Verification items for the finished model (mm, model axes). A direction names the side the tool comes from. Coordinates: 2 decimals unless noted, no trailing zeros. Order: outer loops, then holes, each group sorted by start corner. A loop starts at its lowest first (then second) coordinate and runs counter-clockwise, first axis right, second up. Notation, with made-up numbers: (-10.75, -9.5) -> (39.25, -9.5) arc R24 ccw to (39.25, 15.5) -> close; hole circle Ø3 at (-30, 2). An arc over 180 degrees is marked (long way). Write item = value, one per line. Start each with the question number.
1. Cross-section at C-C on z = 40.5. Record the cut outline in (x, y) (3 decimals).
2. Cross-section at B-B on z = 15.5. Record the cut outline in (x, y), plus the area to 3 significant figures.
3. Cross-section at A-A on y = -50.8. Record the cut outline in (x, z) (3 decimals).
4. Set-up check for faces 4 (the cylindrical face through (30.904, -11.269, 7.96)), 5 (the cylindrical face through (92.25, -88.18, 3.13)), 6 (the flat face through (61.925, -50, 32)): record each of +Z, -Z, +X, -X, +Y, -Y from which the full face is reachable in a straight line by a thin tool's end or side.
5. Go/stop test with flat-tipped pins: P1, Ø3, axis at x = 95.5, y = -91, coming from the +Z side; P2, Ø5, axis at y = -46.5, z = 41.5, coming from the +X side; P3, Ø10, axis at y = -50.8, z = 46.355, coming from the -X side; P4, Ø4, axis at y = -50.8, z = 46.355, coming from the -X side. Record where each tip stops, or that it passes through.
6. Thickness scan on line 1 along X through (y, z) = (-76.5, 32); line 2 along X through (y, z) = (-12, 4). Record the ranges inside material, lowest first. Write a range as from..to.
7. Release check for a two-part mould opening along Y. For faces 1 (the flat face through (54.019, -22.536, 44.761)), 2 (the flat face through (26, -50, 9.525)), 3 (the flat face through (92, -90, 6.35)) record: +Y half, -Y half, draft (parallel to the pull), parting line (faces both ways), or undercut.
8. Cross-section at D-D on x = 103. Record the cut outline in (y, z) (3 decimals).
from build123d import *

# Parameters (mm, degrees)
F1_DEPTH       = 101.6
F3_D           = 4.7752
F3_CBORE_D     = 9.525
F3_CBORE_DEPTH = 3.175
F5_D           = 4.7752
F5_CBORE_D     = 9.525
F5_CBORE_DEPTH = 3.175
F7_D           = 6.35
F8_SIZE        = 44.45
F9_R           = 12.7


with BuildPart() as f1:
    # F0 (on Front) → F1 (new body)
    with BuildSketch(Plane.XZ):
        Polygon((0, 9.525), (0, 0), (119.0752, 0), (119.0752, 9.525), (68.2752, 9.525), (68.2752, 66.675), (61.9252, 66.675), (61.9252, 9.525), (57.15, 9.525), (57.15, 66.675), (50.8, 66.675), (50.8, 9.525), align=None)
    extrude(amount=F1_DEPTH)

    # F3 (through all)
    with Locations(Plane.XY.offset(9.525)):
        with Locations((26.361667, -12.7), (26.361667, -88.9)):
            CounterBoreHole(F3_D / 2, F3_CBORE_D / 2, F3_CBORE_DEPTH)

    # F5 (through all)
    with Locations(Plane.XY.offset(9.525)):
        with Locations((94.527818, -12.7), (94.527818, -88.9)):
            CounterBoreHole(F5_D / 2, F5_CBORE_D / 2, F5_CBORE_DEPTH)

    # F7 (through all)
    with Locations(Plane(origin=(50.8, 0, 0), x_dir=(0, -1, 0), z_dir=(-1, 0, 0))):
        with Locations((50.8, 46.355)):
            Hole(F7_D / 2)

    # F8
    f8_edges = [f1.edges().sort_by_distance(p)[0] for p in [
        (53.975, 0, 66.675),
        (53.975, -101.6, 66.675),
        (65.1002, 0, 66.675),
        (65.1002, -101.6, 66.675),
    ]]
    chamfer(f8_edges, length=F8_SIZE)

    # F9
    f9_edges = [f1.edges().sort_by_distance(p)[0] for p in [
        (0, 0, 4.7625),
        (0, -101.6, 4.7625),
        (119.0752, -101.6, 4.7625),
        (119.0752, 0, 4.7625),
    ]]
    fillet(f9_edges, radius=F9_R)


solid = f1.part
Worked out:
q1.outline = (50.8, -83.325) -> (57.15, -83.325) -> (57.15, -18.275) -> (50.8, -18.275) -> close; (61.925, -83.325) -> (68.275, -83.325) -> (68.275, -18.275) -> (61.925, -18.275) -> close
q2.outline = (50.8, -101.6) -> (57.15, -101.6) -> (57.15, 0) -> (50.8, 0) -> close; (61.93, -101.6) -> (68.28, -101.6) -> (68.28, 0) -> (61.93, 0) -> close
q2.area = 1,290 mm²
q3.outline = (0, 0) -> (119.075, 0) -> (119.075, 9.525) -> (68.275, 9.525) -> (68.275, 43.18) -> (61.925, 43.18) -> (61.925, 9.525) -> (57.15, 9.525) -> (57.15, 43.18) -> (50.8, 43.18) -> (50.8, 9.525) -> (0, 9.525) -> close; (50.8, 49.53) -> (57.15, 49.53) -> (57.15, 66.675) -> (50.8, 66.675) -> close; (61.925, 49.53) -> (68.275, 49.53) -> (68.275, 66.675) -> (61.925, 66.675) -> close
q4.face_4 = +Z
q4.face_5 = +Z, -Z
q4.face_6 = +Z, +Y, -Y
q5.P1 = 6.35
q5.P2 = 68.28
q5.P3 = 50.8
q5.P4 = through
q6.line_1 = 50.8..57.15, 61.93..68.28
q6.line_2 = 0.02..24.08, 28.64..92.25, 96.81..119.06
q7.face_1 = +Y half
q7.face_2 = draft
q7.face_3 = undercut
q8.outline = (-101.6, 0) -> (0, 0) -> (0, 9.525) -> (-101.6, 9.525) -> close
